For this review, take the finished solid that the model builds, in its own axes (mm). Face numbers are marked on the shaded views. A direction names the side the tool comes from. Round coordinates to 2 decimals unless told otherwise and drop trailing zeros. Order: outer loops, then holes, each group sorted by start corner. A loop starts at its lowest first (then second) coordinate and runs counter-clockwise, first axis right, second up. Notation, with made-up numbers: (-31.5, -37.75) - (9.5, -37.75) arc R17 ccw to (9.5, -25.75) - close; hole circle Ø5 at (-34, -3.75). An arc over 180 degrees is marked (long way). One line per item, written item: value.
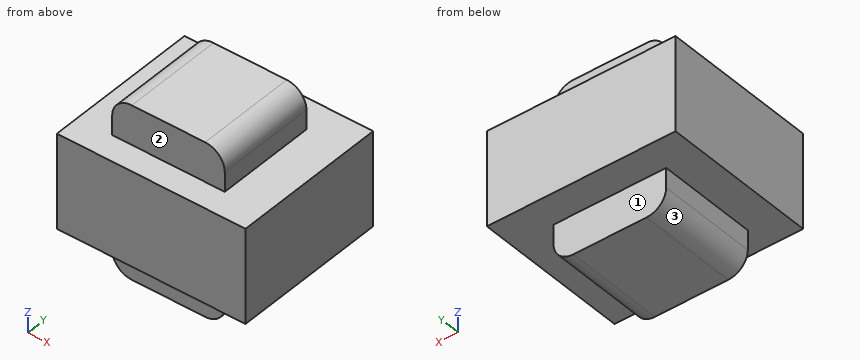
```python
from build123d import *

# Parameters (mm, degrees)
F0_W          = 48
F0_H          = 40
F1_DEPTH      = 24
F2_W          = 28.65385
F2_H          = 25.576925
F3_DEPTH      = 10
F3_DEPTH_BACK = 34
F4_R          = 5


with BuildPart() as f1:
    # F0 (on Top) → F1 (new body)
    with BuildSketch(Plane.XY):
        with Locations((13.115388, -8.846156)):
            Rectangle(F0_W, F0_H)
    extrude(amount=F1_DEPTH)

    # F2 (on face) → F3 (join, two sides)
    with BuildSketch(Plane.XY.offset(24)) as f3_sk:
        with Locations((12.21154, -9.519231)):
            Rectangle(F2_W, F2_H)
    extrude(amount=F3_DEPTH)
    extrude(f3_sk.sketch, amount=-F3_DEPTH_BACK)

    # F4
    f4_edges = [f1.edges().sort_by_distance(p)[0] for p in [
        (26.538465, -9.519232, 34),
        (26.538465, -9.519232, -10),
        (-2.115385, -9.519232, -10),
        (-2.115385, -9.519232, 34),
    ]]
    fillet(f4_edges, radius=F4_R)


solid = f1.part
```
Item 1: Take a section at C-C (z = -2.5). Write out the cut boundary in (x, y).
Returned:
outline: (-2.12, -22.31) - (26.54, -22.31) - (26.54, 3.27) - (-2.12, 3.27) - close
Item 2: Wall thickness on line 1 (Z direction, x = 32, y = 8); line 2 (Y direction, x = 6.5, z = -1); line 3 (X direction, y = 0, z = -1): over which ranges is each line inside the solid? List them lowest first.
Returned:
line 1: 0 to 24
line 2: -22.31 to 3.27
line 3: -2.12 to 26.54
Item 3: Take a section at D-D (x = -4). Write out the cut boundary in (y, z), plus the area to 3 significant figures.
Returned:
outline: (-28.85, 0) - (11.15, 0) - (11.15, 24) - (-28.85, 24) - close
area: 960 mm^2
Item 4: For P1, Ø2.5, axis at y = -14, z = 26.5, coming from the -X side; P2, Ø1.5, axis at y = -3.5, z = 26, coming from the +X side; P3, Ø5, axis at x = 6, z = 30, coming from the -Y side, all flat-tipped, find the tip position at first contact; note any pin that passes through.
Returned:
P1: x = -2.12
P2: x = 26.54
P3: y = -22.31
Item 5: Machinability: for the marked faces 1, 2 and 3, which of the approach directions +Z, -Z, +X, -X, +Y, -Y give a long, thin tool a straight path to every point of the face, cutting with its end or side? Answer none if there is none.
Returned:
face 1: -Z, +X, -X, +Y
face 2: +Z, +X, -X, -Y
face 3: -Z, -X, +Y, -Y
Item 6: Take a section at B-B (y = -12.5). Write out the cut boundary in (x, z), plus the area to 3 significant figures.
Returned:
outline: (-10.88, 0) - (-2.12, 0) - (-2.12, -5) arc R5 ccw to (2.88, -10) - (21.54, -10) arc R5 ccw to (26.54, -5) - (26.54, 0) - (37.12, 0) - (37.12, 24) - (26.54, 24) - (26.54, 29) arc R5 ccw to (21.54, 34) - (2.88, 34) arc R5 ccw to (-2.12, 29) - (-2.12, 24) - (-10.88, 24) - close
area: 1,700 mm^2
Item 7: Take a section at A-A (x = 18). Write out the cut boundary in (y, z).
Returned:
outline: (-28.85, 0) - (-22.31, 0) - (-22.31, -10) - (3.27, -10) - (3.27, 0) - (11.15, 0) - (11.15, 24) - (3.27, 24) - (3.27, 34) - (-22.31, 34) - (-22.31, 24) - (-28.85, 24) - close
